For this review, take the finished solid that the model builds, in its own axes (mm). Give positions to 0.01 mm unless a question says otherwise; leave off trailing zeros. Loops run counter-clockwise (first coordinate to the right, second up) from the corner with the lowest first, then second, coordinate; pieces in that order, holes last.
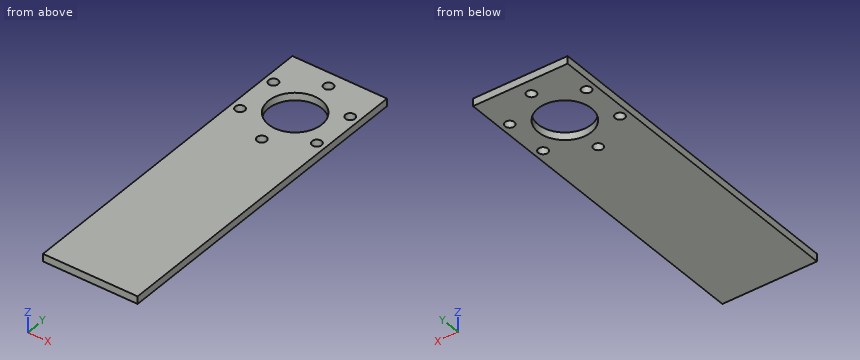
```python
from build123d import *

# Parameters (mm, degrees)
SKETCH2_W              = 50.8
SKETCH2_H              = 177.8
SKETCH2_R              = 14.2875
BOSS_EXTRUDE1_DEPTH    = 4.064
F_10_CLEARANCE_HOLE1_D = 5.1054


with BuildPart() as part:
    # Sketch2 → Boss-Extrude1 (new body)
    with BuildSketch(Plane.XY):
        with Locations((25.4, 88.9)):
            Rectangle(SKETCH2_W, SKETCH2_H)
        with Locations((25.4, 146.05)):
            Circle(SKETCH2_R, mode=Mode.SUBTRACT)
    extrude(amount=BOSS_EXTRUDE1_DEPTH)

    # #10 Clearance Hole1 (through all)
    with Locations(Plane.XY.offset(4.064)):
        with Locations((46.022229928, 157.95625), (25.4, 169.8625), (4.777770072, 157.95625), (4.777770072, 134.14375), (25.4, 122.2375), (46.022229928, 134.14375)):
            Hole(F_10_CLEARANCE_HOLE1_D / 2)


solid = part.part
```
Item 1: Take a section at B-B on x = 25.4. Give the boundary of the cut face in (y, z), and give its area (3 significant figures).
Answer:
outline: (0, 0) - (119.68, 0) - (119.68, 4.06) - (0, 4.06) - close; (124.79, 0) - (131.76, 0) - (131.76, 4.06) - (124.79, 4.06) - close; (160.34, 0) - (167.31, 0) - (167.31, 4.06) - (160.34, 4.06) - close; (172.42, 0) - (177.8, 0) - (177.8, 4.06) - (172.42, 4.06) - close
area: 565 mm2
Item 2: For L1, parallel to Y at x = 25.4, z = 3.1; L2, parallel to Y at x = 4, z = 0.5; L3, parallel to X at y = 155, z = 3.6, list the stretches that pass through material, from the lowest coordinate up.
Answer:
L1: y = 0 to 119.68, 124.79 to 131.76, 160.34 to 167.31, 172.42 to 177.8
L2: y = 0 to 131.71, 136.58 to 155.52, 160.39 to 177.8
L3: x = 0 to 14.26, 36.54 to 50.8
Item 3: Take a section at A-A on y = 146.05. Give the boundary of the cut face in (x, z).
Answer:
outline: (0, 0) - (11.11, 0) - (11.11, 4.06) - (0, 4.06) - close; (39.69, 0) - (50.8, 0) - (50.8, 4.06) - (39.69, 4.06) - close
Item 4: Take a section at C-C on x = 32.5. Give the boundary of the cut face in (y, z), and give its area (3 significant figures).
Answer:
outline: (0, 0) - (133.65, 0) - (133.65, 4.06) - (0, 4.06) - close; (158.45, 0) - (177.8, 0) - (177.8, 4.06) - (158.45, 4.06) - close
area: 622 mm2
Item 5: Clearance check with a flat-ended pin moving along its axis: pin 1 Ø4 at (x, y) = (4.78, 157.96) entering from +Z. State where the tip first meets the part, or that it passes through.
Answer:
pin 1: passes through
Item 6: Take a section at D-D on z = 2.8. State how many separate pieces and enclosed holes the cut face has, and give its area (3 significant figures).
Answer:
separate pieces: 1
enclosed holes: 7
area: 8,270 mm2
